Check sheet for the modelled part. Datum: model origin and axes. Units: mm. A direction names the side the tool comes from. Round coordinates to 2 decimals unless told otherwise and drop trailing zeros. Write each loop counter-clockwise with the first axis right and the second up, starting at its lowest first coordinate (ties: lowest second). Pieces come first, ordered by that corner, then holes.
Item 1: Depth check by flat-ended pin: pin 1 (1.5 mm diameter, centred on x = 57, z = 2, fed in from -Y); pin 2 (0.9 mm diameter, centred on x = 5.5, z = 2, fed in from -Y); pin 3 (1.5 mm diameter, centred on y = -1.5, z = 1, fed in from +X). Enter the tip coordinate at first touch or a pass-through.
Item 2: Section check B-B, the plane x = 28. Record the cut outline in (y, z).
Item 3: Section check A-A, the plane y = 5. Record the cut outline in (x, z).
Item 4: Release check for a two-part mould opening along X. For faces 1 (the flat face through (90, -3, 1)), 2 (the flat face through (59, 0, 1)), 3 (the flat face through (112.3, 3, 1)) record: pulls with the +X half, pulls with the -X half, needs draft (parallel to the pull), parting line crosses it, or undercut.
Item 5: Material ranges on line 1 along X through (y, z) = (19, 2.9); line 2 along Y through (x, z) = (27, 0.65); line 3 along Y through (x, z) = (69.5, 0.7), recorded low to high.
Item 6: Set-up check for faces 4 (the flat face through (41.5, -2, 1)), 5 (the flat face through (6.5, 4, 1)), 6 (the flat face through (21.4, 12, 1)): record each of +Z, -Z, +X, -X, +Y, -Y from which the full face is reachable in a straight line by a thin tool's end or side.
Item 7: Section check C-C, the plane z = 2.55. Record the cut outline in (x, y), plus the area to 3 significant figures.
Item 8: Section check D-D, the plane x = 68.5. Record the cut outline in (y, z).
from build123d import *

# Parameters (mm, degrees)
EXTRUDE_1_DEPTH = 3


with BuildPart() as part:
    # 草图2 → 凸台-拉伸1 (new body)
    with BuildSketch(Plane.XY):
        Polygon((41.5, 0), (59.4, 0), (77.3, 0), (77.3, -3), (102.3, -3), (102.3, 0), (112.3, 0), (112.3, 7), (115.3, 7), (115.3, 23), (112.3, 23), (112.3, 30), (6.5, 30), (6.5, 23), (3.5, 23), (3.5, 7), (6.5, 7), (6.5, 0), (16.5, 0), (16.5, -3), (41.5, -3), align=None)
        Polygon((26.4, 4), (21.4, 4), (21.4, 20), (26.4, 20), (31.4, 20), (31.4, 4), align=None, mode=Mode.SUBTRACT)
    extrude(amount=EXTRUDE_1_DEPTH)


solid = part.part
Values found:
1. pin 1: stops at y = 0
1. pin 2: stops at y = 7
1. pin 3: stops at x = 102.3
2. outline: (-3, 0) - (4, 0) - (4, 3) - (-3, 3) - close; (20, 0) - (30, 0) - (30, 3) - (20, 3) - close
3. outline: (6.5, 0) - (21.4, 0) - (21.4, 3) - (6.5, 3) - close; (31.4, 0) - (112.3, 0) - (112.3, 3) - (31.4, 3) - close
4. face 1: needs draft
4. face 2: undercut
4. face 3: pulls with the +X half
5. line 1: x = 3.5 to 21.4, 31.4 to 115.3
5. line 2: y = -3 to 4, 20 to 30
5. line 3: y = 0 to 30
6. face 4: +Z, -Z, -Y
6. face 5: +Z, -Z, -X, -Y
6. face 6: +Z, -Z
7. outline: (3.5, 7) - (6.5, 7) - (6.5, 0) - (16.5, 0) - (16.5, -3) - (41.5, -3) - (41.5, 0) - (77.3, 0) - (77.3, -3) - (102.3, -3) - (102.3, 0) - (112.3, 0) - (112.3, 7) - (115.3, 7) - (115.3, 23) - (112.3, 23) - (112.3, 30) - (6.5, 30) - (6.5, 23) - (3.5, 23) - close; hole (21.4, 4) - (31.4, 4) - (31.4, 20) - (21.4, 20) - close
7. area: 3,260 mm2
8. outline: (0, 0) - (30, 0) - (30, 3) - (0, 3) - close
